Read the model definition and answer for the solid it produces. Units are mm, in the model's axes. Coordinates: 2 decimals unless noted, no trailing zeros. Loops run counter-clockwise (first coordinate to the right, second up) from the corner with the lowest first, then second, coordinate; pieces in that order, holes last. Notation, with made-up numbers: (36, 50) -> (60, 50) arc R24 ccw to (60, 85) -> close; hole circle Ø11 at (27.5, -24). An arc over 180 degrees is marked (long way). Answer as a JSON object with one key per item and string values. Group by question number.
Q1. The part is cut by section A-A on z = 0. Write down the section's boundary in (x, y) (3 decimals).
Q2. Straight lines are drawn through the part: line 1 along Y through (x, z) = (-46.5, -16); line 2 along Z through (x, y) = (18, 4.5); line 3 along X through (y, z) = (11.25, 14). For each, find the intervals that lie inside material, in ascending order. Write a range as [from, to].
Q3. Each of these flat-tipped pins is pushed along its axis until it touches: P1, Ø4, axis at y = 6, z = -32.5, coming from the -X side; P2, Ø2, axis at x = -57, z = 19.5, coming from the +Y side; P3, Ø2, axis at x = -7, y = 5.5, coming from the -Z side. Where does it stop, or does it pass through?
Q4. The part is cut by section C-C on y = 15.75. Write down the section's boundary in (x, z).
Q5. The part is cut by section D-D on y = 4. Write down the section's boundary in (x, z) (3 decimals), and give its area (3 significant figures).
Q6. The part is cut by section B-B on x = 0. Write down the section's boundary in (y, z) (3 decimals), and give its area (3 significant figures).
from build123d import *

# Parameters (mm, degrees)
F0_R     = 73.025
F1_DEPTH = 12.7
F2_R     = 5.08
F3_R     = 12.7
F4_DEPTH = 6.35


with BuildPart() as f1:
    # F0 (on Front) → F1 (new body)
    with BuildSketch(Plane.XZ):
        Circle(F0_R)
    extrude(amount=-F1_DEPTH)

    # F2
    f2_edges = [f1.edges().sort_by_distance(p)[0] for p in [
        (-73.025, 12.7, 0),
    ]]
    fillet(f2_edges, radius=F2_R)

    # F3 (on face) → F4 (join)
    with BuildSketch(Plane(origin=(0, 12.7, 0), x_dir=(-1, 0, 0), z_dir=(0, 1, 0))):
        with Locations((48.768654, 0)):
            Circle(F3_R)
    extrude(amount=F4_DEPTH)


solid = f1.part
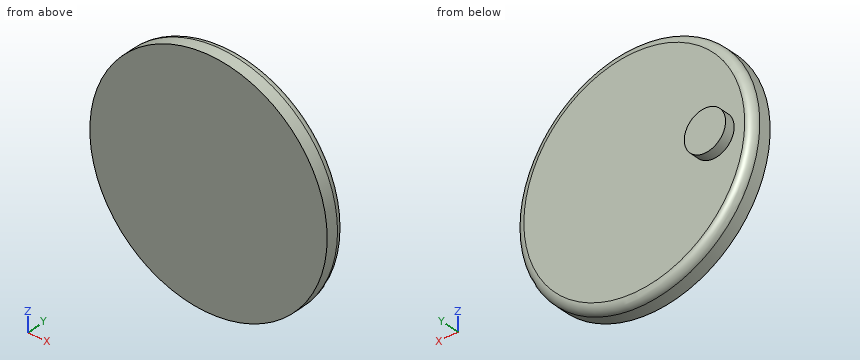
Final values:
{
 "1": {"outline": "(-73.025, 0) -> (73.025, 0) -> (73.025, 7.62) arc R5.08 ccw to (67.945, 12.7) -> (-36.069, 12.7) -> (-36.069, 19.05) -> (-61.469, 19.05) -> (-61.469, 12.7) -> (-67.945, 12.7) arc R5.08 ccw to (-73.025, 7.62) -> close"},
 "2": {"line 1": "y = [0, 12.7]", "line 2": "z = [-70.77, 70.77]", "line 3": "x = [-70.11, 70.11]"},
 "3": {"P1": "stops at x = -66.35", "P2": "stops at y = 12.7", "P3": "stops at z = -72.78"},
 "4": {"outline": "circle Ø25.4 at (-48.77, 0)"},
 "5": {"outline": "circle Ø146.05 at (0, 0)", "area": "16,800 mm2"},
 "6": {"outline": "(0, -73.025) -> (7.62, -73.025) arc R5.08 ccw to (12.7, -67.945) -> (12.7, 67.945) arc R5.08 ccw to (7.62, 73.025) -> (0, 73.025) -> close", "area": "1,840 mm2"}
}
